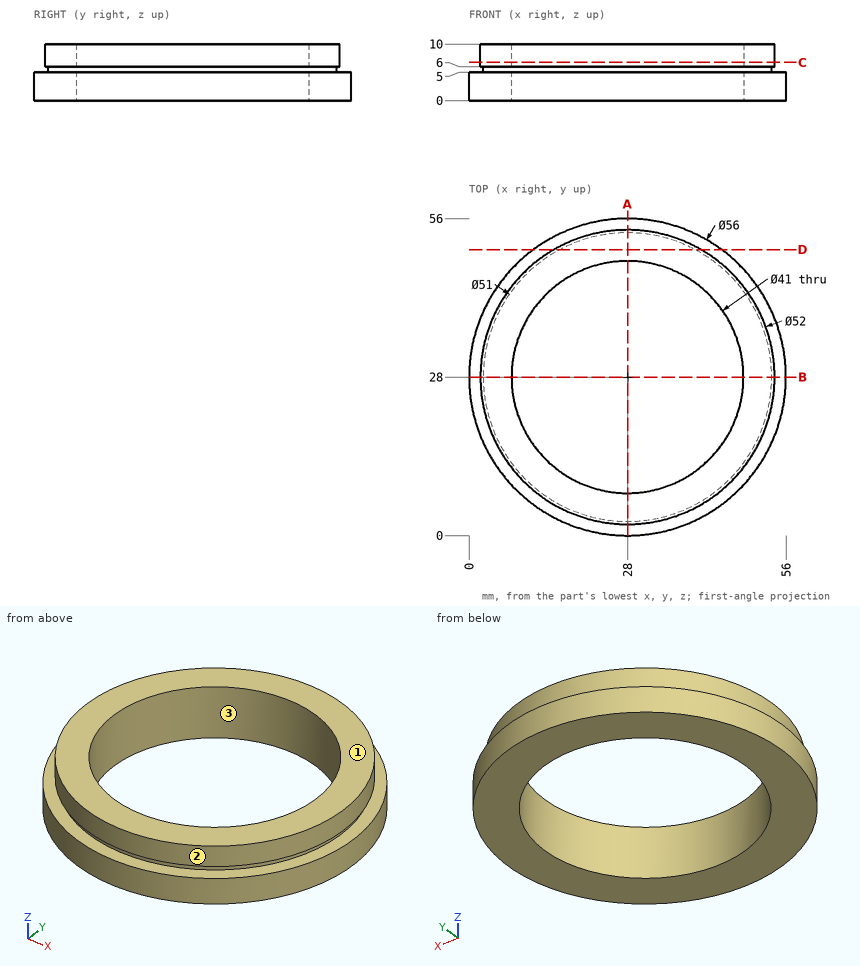
Check sheet for the drawn part. Datum: minimum x, y, z corner. Units: mm. Coordinates: 2 decimals unless noted, no trailing zeros. Write each loop counter-clockwise with the first axis right and the second up, starting at its lowest first coordinate (ties: lowest second). Pieces come first, ordered by that corner, then holes. Notation, with made-up numbers: M -0.75,-12 L 27.25,-12 A20 ccw 27.25,24 Z; hole C 66.25,31 d8. An arc over 180 degrees is marked long. Use a Markdown table: item, result.
Q1. Thickness scan on line 1 (Y direction, x = 28, z = 6.5); line 2 (Z direction, x = 12, y = 8); line 3 (Z direction, x = 43, y = 6.5). Record the ranges inside material, lowest first.
Reply:
| item | result |
|---|---|
| line 1 | y = 2 to 7.5, 48.5 to 54 |
| line 2 | z = 0 to 5, 6 to 10 |
| line 3 | z = 0 to 5 |
Q2. Sectioned sample at C-C, the plane z = 6.75. Record the boundary of the cut face in (x, y).
Reply:
| item | result |
|---|---|
| outline | C 28,28 d52; hole C 28,28 d41 |
Q3. Draft check along Y on the marked faces 1, 2 and 3. Enter one of: +Y half, -Y half, draft (parallel to the pull), parting line (faces both ways), or undercut.
Reply:
| item | result |
|---|---|
| face 1 | draft |
| face 2 | parting line |
| face 3 | undercut |
Q4. Go/stop test with flat-tipped pins: P1, Ø1, axis at y = 29.5, z = 6, coming from the +X side; P2, Ø10, axis at x = 28.5, y = 17.5, coming from the +Z side; P3, Ø2, axis at y = 16, z = 1.5, coming from the +X side. Record where each tip stops, or that it passes through.
Reply:
| item | result |
|---|---|
| P1 | stops at x = 53.98 |
| P2 | passes through |
| P3 | stops at x = 53.75 |
Q5. Sectioned sample at A-A, the plane x = 28. Record the boundary of the cut face in (y, z).
Reply:
| item | result |
|---|---|
| outline | M 0,0 L 7.5,0 L 7.5,10 L 2,10 L 2,6 L 2.5,6 L 2.5,5 L 0,5 Z; M 48.5,0 L 56,0 L 56,5 L 53.5,5 L 53.5,6 L 54,6 L 54,10 L 48.5,10 Z |
Q6. Sectioned sample at D-D, the plane y = 50.5. Record the boundary of the cut face in (x, z).
Reply:
| item | result |
|---|---|
| outline | M 11.33,0 L 44.67,0 L 44.67,5 L 40,5 L 40,6 L 41.03,6 L 41.03,10 L 14.97,10 L 14.97,6 L 16,6 L 16,5 L 11.33,5 Z |
